from build123d import *

# Parameters (mm, degrees)
SKETCH1_R               = 3
BOSS_EXTRUDE1_DEPTH     = 252
CUT_EXTRUDE2_DEPTH      = 253.035711755
CUT_EXTRUDE2_DEPTH_BACK = 253.035711755
SKETCH2_W               = 2
SKETCH2_H               = 17.5


with BuildPart() as part:
    # Sketch1 → Boss-Extrude1 (new body)
    with BuildSketch(Plane(origin=(0, 0, 0), x_dir=(1, 0, 0), z_dir=(0, 1, 0))):
        with Locations(Location((0, 0, 0), (0, 0, 270))):
            Circle(SKETCH1_R)
    extrude(amount=BOSS_EXTRUDE1_DEPTH)

    # Sketch2 → Cut-Extrude2 (cut, two sides: drawn at the far end of the back side and taken through both)
    with BuildSketch(Plane(origin=(0, 0, 0), x_dir=(0, 0, -1), z_dir=(1, 0, 0)).offset(-CUT_EXTRUDE2_DEPTH_BACK)):
        with Locations((0, 243.25)):
            Rectangle(SKETCH2_W, SKETCH2_H)
        with Locations((0, 8.75)):
            Rectangle(SKETCH2_W, SKETCH2_H)
    extrude(amount=CUT_EXTRUDE2_DEPTH + CUT_EXTRUDE2_DEPTH_BACK, mode=Mode.SUBTRACT)


solid = part.part
Input: part model. Units: mm. Frame: model coordinates. A direction names the side the tool comes from. Coordinates: 2 decimals unless noted, no trailing zeros. Order: outer loops, then holes, each group sorted by start corner. A loop starts at its lowest first (then second) coordinate and runs counter-clockwise, first axis right, second up. Notation, with made-up numbers: M 6.25,7 L 41.25,7 A19 cw 41.25,43 Z; hole C 63,-30.75 d10. An arc over 180 degrees is marked long. One line per question, with ' | ' between items.
Item 1: Ray query, line 1 along Y through (x, z) = (-2.4, -0.9); line 2 along Z through (x, y) = (-0.1, 237.5); line 3 along X through (y, z) = (197.5, 1.05). Return the intervals inside material, ascending.
Geometry results:
line 1: y = 17.5 to 234.5 | line 2: z = -3 to -1, 1 to 3 | line 3: x = -2.81 to 2.81
Item 2: Section B-B (y = 125). Output: boundary loops of the cut face in (x, z), then the cut area to 3 significant figures.
Geometry results:
outline: C 0,0 d6 | area: 28.3 mm^2
Item 3: Pin query (flat end, axial travel): pin 1 (1.6 mm diameter, centred on x = -1, z = 0, fed in from +Y); pin 2 (1.7 mm diameter, centred on x = 1.5, y = 246.5, fed in from +Z); pin 3 (1 mm diameter, centred on x = -1, z = 0, fed in from -Y). Return the tip coordinate at first contact, or that it passes through.
Geometry results:
pin 1: stops at y = 234.5 | pin 2: stops at z = 2.93 | pin 3: stops at y = 17.5
Item 4: Section A-A (x = 0). Output: boundary loops of the cut face in (y, z), then the cut area to 3 significant figures.
Geometry results:
outline: M 0,-3 L 252,-3 L 252,-1 L 234.5,-1 L 234.5,1 L 252,1 L 252,3 L 0,3 L 0,1 L 17.5,1 L 17.5,-1 L 0,-1 Z | area: 1,440 mm^2
Item 5: Section C-C (z = 0). Output: boundary loops of the cut face in (x, y).
Geometry results:
outline: M -3,17.5 L 3,17.5 L 3,234.5 L -3,234.5 Z
Item 6: Reachability of faces 1 (the cylindrical face through (-1.15, 124.24, 2.77)), 2 (the flat face through (0, 9, -1)), 3 (the flat face through (0, 243, -1)) from +Z, -Z, +X, -X, +Y, -Y: full face, straight path, thin tool, end or side. Return the list, or none.
Geometry results:
face 1: +Y, -Y | face 2: +X, -X, -Y | face 3: +X, -X, +Y
